from build123d import *

# Parameters (mm, degrees)
ESQUISSE1_W                                        = 18
ESQUISSE1_H                                        = 36
BOSS_EXTRU_1_DEPTH                                 = 7
CHAMBRAGE_POUR_VIS_T_TE_HEXAGONALE_M41_D           = 4.5
CHAMBRAGE_POUR_VIS_T_TE_HEXAGONALE_M41_CBORE_D     = 8
CHAMBRAGE_POUR_VIS_T_TE_HEXAGONALE_M41_CBORE_DEPTH = 4.4


with BuildPart() as part:
    # Esquisse1 → Boss.-Extru.1 (new body, symmetric)
    with BuildSketch(Plane.XY):
        Rectangle(ESQUISSE1_W, ESQUISSE1_H)
    extrude(amount=BOSS_EXTRU_1_DEPTH, both=True)

    # Chambrage pour vis à tête hexagonale M41 (through all)
    with Locations(Plane(origin=(0, 0, -7), x_dir=(-1, 0, 0), z_dir=(0, 0, -1))):
        with Locations((0, 8.5), (0, -8.5)):
            CounterBoreHole(CHAMBRAGE_POUR_VIS_T_TE_HEXAGONALE_M41_D / 2, CHAMBRAGE_POUR_VIS_T_TE_HEXAGONALE_M41_CBORE_D / 2, CHAMBRAGE_POUR_VIS_T_TE_HEXAGONALE_M41_CBORE_DEPTH)


solid = part.part
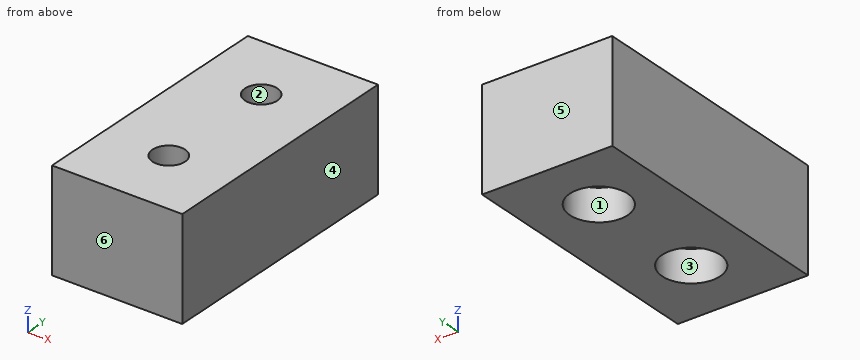
Input: part model. Units: mm. Frame: model coordinates. Face numbers are marked on the shaded views. A direction names the side the tool comes from. Give positions to 0.01 mm unless a question says otherwise; leave off trailing zeros. Loops run counter-clockwise (first coordinate to the right, second up) from the corner with the lowest first, then second, coordinate; pieces in that order, holes last. Notation, with made-up numbers: (62, 16) - (121, 16) arc R12 ccw to (121, 22) - close; hole circle Ø7 at (1.5, 52.5). An arc over 180 degrees is marked (long way). Use CSV: the item, a comma, the result in double quotes. Start each with the question number.
Item 1: Reachability of the marked faces 1 and 2 from +Z, -Z, +X, -X, +Y, -Y: full face, straight path, thin tool, end or side. Return the list, or none.
Item 2: Section C-C on z = 4.75. Return loops of the section in (x, y), then the cut area to 3 significant figures.
Item 3: Section D-D on x = -3.5. Return loops of the section in (y, z).
Item 4: Contact query for a flat-ended pin moving along its axis: P1, Ø2.5, axis at x = 1.5, y = 10, coming from the -Z side. Output: stop coordinate, or through.
Item 5: Section A-A on y = 8.5. Return loops of the section in (x, z), then the cut area to 3 significant figures.
Item 6: Line query: line 1 (Y direction, x = 0, z = 3.25); line 2 (Y direction, x = 0, z = -4.1); line 3 (X direction, y = -9.5, z = 3.25). Output: solid intervals per line, ascending.
Item 7: Section B-B on x = 0. Return loops of the section in (y, z), then the cut area to 3 significant figures.
Item 8: Mould query, pull axis Y, two halves, no side actions, for the marked faces 3, 4, 5 and 6. Classes: pulls with the +Y half, pulls with the -Y half, needs draft (parallel to the pull), parting line crosses it, or undercut.
Ans:
1,face 1,"-Z"
1,face 2,"+Z, -Z"
2,outline,"(-9, -18) - (9, -18) - (9, 18) - (-9, 18) - close; hole circle Ø4.5 at (0, -8.5); hole circle Ø4.5 at (0, 8.5)"
2,area,"616 mm2"
3,outline,"(-18, -7) - (-10.44, -7) - (-10.44, -2.6) - (-6.56, -2.6) - (-6.56, -7) - (6.56, -7) - (6.56, -2.6) - (10.44, -2.6) - (10.44, -7) - (18, -7) - (18, 7) - (-18, 7) - close"
4,P1,"stops at z = -2.6"
5,outline,"(-9, -7) - (-4, -7) - (-4, -2.6) - (-2.25, -2.6) - (-2.25, 7) - (-9, 7) - close; (2.25, -2.6) - (4, -2.6) - (4, -7) - (9, -7) - (9, 7) - (2.25, 7) - close"
5,area,"174 mm2"
6,line 1,"y = -18 to -10.75, -6.25 to 6.25, 10.75 to 18"
6,line 2,"y = -18 to -12.5, -4.5 to 4.5, 12.5 to 18"
6,line 3,"x = -9 to -2.02, 2.02 to 9"
7,outline,"(-18, -7) - (-12.5, -7) - (-12.5, -2.6) - (-10.75, -2.6) - (-10.75, 7) - (-18, 7) - close; (-6.25, -2.6) - (-4.5, -2.6) - (-4.5, -7) - (4.5, -7) - (4.5, -2.6) - (6.25, -2.6) - (6.25, 7) - (-6.25, 7) - close; (10.75, -2.6) - (12.5, -2.6) - (12.5, -7) - (18, -7) - (18, 7) - (10.75, 7) - close"
7,area,"347 mm2"
8,face 3,"undercut"
8,face 4,"needs draft"
8,face 5,"pulls with the +Y half"
8,face 6,"pulls with the -Y half"
